Build history of the part. All positions in model axes, mm. A direction names the side the tool comes from. Round coordinates to 2 decimals unless told otherwise and drop trailing zeros. Write each loop counter-clockwise with the first axis right and the second up, starting at its lowest first coordinate (ties: lowest second). Pieces come first, ordered by that corner, then holes.
Autodesk Inventor part; units mm, degrees
ref_plane "YZ Plane" through (0, 0, 0) normal (1, 0, 0) x (0, 1, 0)
ref_plane "XZ Plane" through (0, 0, 0) normal (0, 1, 0) x (-1, 0, 0)
ref_plane "XY Plane" through (0, 0, 0) normal (0, 0, 1) x (1, 0, 0)
sketch "Sketch5" plane through (0, 0, 0) normal (0, 0, 1) x (1, 0, 0)
  line L0 (-42.5, 97.5) -> (42.5, 97.5)
  line L1 (42.5, 97.5) -> (42.5, -97.5)
  line L2 (42.5, -97.5) -> (-42.5, -97.5)
  line L3 (-42.5, -97.5) -> (-42.5, 97.5)
  point P0 (0, 0)
  point P1 (0, 97.5)
  point P2 (42.5, 0)
  point P3 (-42.5, 0)
  dimension "d8" = 195
  dimension "d9" = 85
extrude "Extrusion5" add sketch "Sketch5" along normal mid plane 15
sketch "Sketch6" plane through (0, 0, 7.5) normal (0, 0, 1) x (1, 0, 0)
  line L0 (42.5, -97.5) -> (16.5, -97.5)
  line L1 (16.5, -97.5) -> (16.5, -9.5)
  line L2 (16.5, -9.5) -> (42.5, -9.5)
  line L3 (42.5, -9.5) -> (42.5, -97.5)
  point P0 (0, 0)
  dimension "d12" = 88
  dimension "d13" = 26
extrude "Extrusion6" cut sketch "Sketch6" against normal blind 15
sketch "Sketch7" plane through (0, 0, -7.5) normal (0, 0, -1) x (-1, 0, 0)
  line L0 (42.5, 97.5) -> (-42.5, 97.5)
  circle A0 centre (-31.5, 83.75) radius 4.25
  circle A1 centre (-31.5, 43.75) radius 4.25
  circle A2 centre (-31.5, 3.75) radius 4.25
  circle A3 centre (-6.5, -82.5) radius 4.25
  circle A4 centre (33.5, -82.5) radius 4.25
  line L1 (42.5, -97.5) -> (42.5, 97.5)
  line L2 (-16.5, -9.5) -> (-16.5, -97.5)
  point P0 (0, 0)
  dimension "d18" = 8.5
  dimension "d19" = 40
  dimension "d20" = 40
  dimension "d21" = 13.75
  dimension "d22" = 40
  dimension "d66" = 74
  dimension "d68" = 59
  dimension "d70" = 10
hole "Hole1" at (31.5, 83.75, -7.5) at (31.5, 43.75, -7.5) at (31.5, 3.75, -7.5) at (-33.5, -82.5, -7.5) at (6.5, -82.5, -7.5) direction (0, 0, 1) diameter 8.5 end through all counterbore diameter 14 counterbore depth 9
sketch "Sketch9" plane through (-42.5, -97.5, 7.5) normal (-1, 0, 0) x (0, 0, 1)
  circle A0 centre (-7.5, 167.5) radius 3
  circle A1 centre (-7.5, 112.5) radius 3
  circle A2 centre (-7.5, 57.5) radius 3
  line L0 (0, 0) -> (-15, 0)
  point P0 (-7.5, 97.5)
  dimension "d55" = 55
  dimension "d56" = 55
  dimension "d57" = 6
  dimension "d65" = 57.5
hole "Hole3" at (-42.5, -40, 0) at (-42.5, 15, 0) at (-42.5, 70, 0) direction (1, 0, 0) diameter 4.917 depth 15 tip angle 118
equation "\"d20\" = d19"
properties part number "BC-10013" material "Alumínio 7075"
1) Slice it at B-B (y = 3.75). Write the cut outline in (x, z), plus the area to 3 significant figures.
Results:
outline: (-42.5, -7.5) - (24.5, -7.5) - (24.5, 1.5) - (27.25, 1.5) - (27.25, 7.5) - (-42.5, 7.5) - close; (35.75, 1.5) - (38.5, 1.5) - (38.5, -7.5) - (42.5, -7.5) - (42.5, 7.5) - (35.75, 7.5) - close
area: 1,100 mm2
2) Wall check: L1, parallel to Y at x = 31.5, z = 5.8; L2, parallel to Y at x = 31.5, z = -3; L3, parallel to X at y = 83.75, z = -5.5. Give the ranges that are in metal, low to high.
Results:
L1: y = -9.5 to -0.5, 8 to 39.5, 48 to 79.5, 88 to 97.5
L2: y = -9.5 to -3.25, 10.75 to 36.75, 50.75 to 76.75, 90.75 to 97.5
L3: x = -42.5 to 24.5, 38.5 to 42.5
3) Mould opens along X. For faces 1 (the cylindrical face through (31.192, 76.757, -2.937)), 2 (the flat face through (-42.5, -1, 0)), 3 (the flat face through (-1, 97.5, 0)), 4 (the flat face through (16.5, -54, 0)) say: released by +X, released by -X, zero draft, split by the parting line, or undercut.
Results:
face 1: undercut
face 2: released by -X
face 3: zero draft
face 4: released by +X
4) Slice it at D-D (y = -82.5). Write the cut outline in (x, z).
Results:
outline: (-42.5, -7.5) - (-40.5, -7.5) - (-40.5, 1.5) - (-37.75, 1.5) - (-37.75, 7.5) - (-42.5, 7.5) - close; (-29.25, 1.5) - (-26.5, 1.5) - (-26.5, -7.5) - (-0.5, -7.5) - (-0.5, 1.5) - (2.25, 1.5) - (2.25, 7.5) - (-29.25, 7.5) - close; (10.75, 1.5) - (13.5, 1.5) - (13.5, -7.5) - (16.5, -7.5) - (16.5, 7.5) - (10.75, 7.5) - close
5) Pin check, flat tips, straight feed: pin 1 Ø11 at (x, y) = (31.5, 83.75) entering from -Z; pin 2 Ø4.5 at (y, z) = (-40, 0) entering from -X; pin 3 Ø1.5 at (y, z) = (-15.5, -4) entering from +X. Stop position of each tip, or through.
Results:
pin 1: stops at z = 1.5
pin 2: stops at x = -27.37
pin 3: stops at x = 16.5
6) Which spindle directions (+Z, -Z, +X, -X, +Y, -Y) get a long thin tool onto all of the face, cutting with end or side? Do faces 5 (the cylindrical face through (2.286, -83.053, 4.542)), 6 (the cylindrical face through (34.181, 50.216, -2.937)), 7 (the cylindrical face through (-34.89, 72.4, -0.53)). Say none if no direction does.
Results:
face 5: +Z, -Z
face 6: -Z
face 7: -X
7) Slice it at A-A (x = -33.5). Write the cut outline in (y, z).
Results:
outline: (-97.5, -7.5) - (-89.5, -7.5) - (-89.5, 1.5) - (-86.75, 1.5) - (-86.75, 7.5) - (-97.5, 7.5) - close; (-78.25, 1.5) - (-75.5, 1.5) - (-75.5, -7.5) - (97.5, -7.5) - (97.5, 7.5) - (-78.25, 7.5) - close; hole circle Ø4.92 at (-40, 0); hole circle Ø4.92 at (15, 0); hole circle Ø4.92 at (70, 0)
8) Slice it at C-C (x = 31.5). Write the cut outline in (y, z), plus the area to 3 significant figures.
Results:
outline: (-9.5, -7.5) - (-3.25, -7.5) - (-3.25, 1.5) - (-0.5, 1.5) - (-0.5, 7.5) - (-9.5, 7.5) - close; (8, 1.5) - (10.75, 1.5) - (10.75, -7.5) - (36.75, -7.5) - (36.75, 1.5) - (39.5, 1.5) - (39.5, 7.5) - (8, 7.5) - close; (48, 1.5) - (50.75, 1.5) - (50.75, -7.5) - (76.75, -7.5) - (76.75, 1.5) - (79.5, 1.5) - (79.5, 7.5) - (48, 7.5) - close; (88, 1.5) - (90.75, 1.5) - (90.75, -7.5) - (97.5, -7.5) - (97.5, 7.5) - (88, 7.5) - close
area: 1,070 mm2
